Work out the finished part from the listing and answer in its coordinate system (mm). A direction names the side the tool comes from. Round coordinates to 2 decimals unless told otherwise and drop trailing zeros. Order: outer loops, then holes, each group sorted by start corner. A loop starts at its lowest first (then second) coordinate and runs counter-clockwise, first axis right, second up. Notation, with made-up numbers: M 33.5,-10 L 82.5,-10 A25 ccw 82.5,17 Z; hole C 59,62.5 d10. An arc over 180 degrees is marked long. Return JSON: item names as keys, results as strings.
from build123d import *

# Parameters (mm, degrees)
SALIENTE_EXTRUIR1_DEPTH = 1.8
CROQUIS2_W              = 7.6
CROQUIS2_H              = 25
SALIENTE_EXTRUIR2_DEPTH = 0.9
SALIENTE_EXTRUIR3_DEPTH = 3
CORTAR_EXTRUIR1_DEPTH   = 2.05
SALIENTE_EXTRUIR4_DEPTH = 20
REDONDEO1_R             = 2


with BuildPart() as part:
    # Croquis1 → Saliente-Extruir1 (new body)
    with BuildSketch(Plane.XY):
        Polygon((0, 0), (25, 0), (0, -25), align=None)
    extrude(amount=SALIENTE_EXTRUIR1_DEPTH)

    # Croquis2 → Saliente-Extruir2 (add)
    with BuildSketch(Plane.ZY):
        with Locations((-2, -12.5)):
            Rectangle(CROQUIS2_W, CROQUIS2_H)
    extrude(amount=SALIENTE_EXTRUIR2_DEPTH)

    # Croquis3 → Saliente-Extruir3 (add)
    with BuildSketch(Plane(origin=(0, 0, -5.8), x_dir=(-1, 0, 0), z_dir=(0, 0, -1))):
        Polygon((0, 0), (-25, 0), (0, -25), align=None)
    extrude(amount=-SALIENTE_EXTRUIR3_DEPTH)

    # Croquis4 → Cortar-Extruir1 (cut)
    with BuildSketch(Plane.XY.offset(-2.8)):
        Polygon((18.8816387, -4.704147737), (4.704147737, -18.8816387), (0.426151711, -14.603642674), (14.603642674, -0.426151711), align=None)
    extrude(amount=-CORTAR_EXTRUIR1_DEPTH, mode=Mode.SUBTRACT)

    # Croquis5 → Saliente-Extruir4 (add)
    with BuildSketch(Plane.ZY.offset(0.9)):
        Polygon((1.8, 0), (7.8, 0), (9.921320344, -2.121320344), (9.072792206, -2.969848481), (7.302943725, -1.2), (1.8, -1.2), align=None)
    extrude(amount=-SALIENTE_EXTRUIR4_DEPTH)

    # Redondeo1
    redondeo1_edges = [part.edges().sort_by_distance(p)[0] for p in [
        (9.1, 0, 7.8),
        (9.1, -1.2, 7.302943725),
    ]]
    fillet(redondeo1_edges, radius=REDONDEO1_R)


solid = part.part
Item 1: Which of the six approach directions +Z, -Z, +X, -X, +Y, -Y give full straight-line access (tool end or side, diameter ignored) to faces 1 (the flat face through (8.96, -2.386, 8.489)), 2 (the flat face through (0, -12, -1)), 3 (the flat face through (13, -12, -4)), 4 (the flat face through (7.42, -7.61, -3.81))?
Output:
{"face 1": "+X, -X, -Y", "face 2": "+X, +Y, -Y", "face 3": "+Z, -Z, +X, -Y", "face 4": "none"}
Item 2: Find section C-C (y = -21). Determine the outline of the cut face in (x, z).
Output:
{"outline": "M -0.9,-5.8 L 4,-5.8 L 4,-2.8 L 0,-2.8 L 0,0 L 4,0 L 4,1.8 L -0.9,1.8 Z"}
Item 3: Find section D-D (x = 22.75). Determine the outline of the cut face in (y, z), plus the area to 3 significant figures.
Output:
{"outline": "M -2.25,-5.8 L 0,-5.8 L 0,-2.8 L -2.25,-2.8 Z; M -2.25,0 L 0,0 L 0,1.8 L -2.25,1.8 Z", "area": "10.8 mm^2"}
Item 4: Find section A-A (x = 20). Determine the outline of the cut face in (y, z), plus the area to 3 significant figures.
Output:
{"outline": "M -5,-5.8 L 0,-5.8 L 0,-2.8 L -5,-2.8 Z; M -5,0 L 0,0 L 0,1.8 L -5,1.8 Z", "area": "24.0 mm^2"}
Item 5: The mould has two halves that part along Y. Classify faces 5 (the flat face through (19.1, -1, 6)), 6 (the flat face through (11.892, -11.694, -3.811)), 7 (the cylindrical face through (9.24, -0.15, 7.73)): pulls with the +Y half, pulls with the -Y half, needs draft (parallel to the pull), parting line crosses it, or undercut.
Output:
{"face 5": "needs draft", "face 6": "undercut", "face 7": "pulls with the +Y half"}
Item 6: Find section B-B (z = -4.5). Determine the outline of the cut face in (x, y).
Output:
{"outline": "M -0.9,-25 L 0,-25 L 25,0 L -0.9,0 Z; hole M 0.43,-14.6 L 4.7,-18.88 L 18.88,-4.7 L 14.6,-0.43 Z"}
Item 7: Each of these flat-tipped pins is pushed along its axis until it touches: pin 1 (5 mm diameter, centred on x = 4, y = -13, fed in from +Z); pin 2 (1.5 mm diameter, centred on x = 5, z = -3.5, fed in from -Y); pin 3 (12.5 mm diameter, centred on x = 18.5, y = -11, fed in from -Z); pin 4 (2.5 mm diameter, centred on x = 8, z = 4, fed in from -Y). Where does it stop, or does it pass through?
Output:
{"pin 1": "stops at z = 1.8", "pin 2": "stops at y = -20.75", "pin 3": "stops at z = -5.8", "pin 4": "stops at y = -1.2"}
Item 8: Consider line 1 along Z through (x, y) = (1.75, -17.75); line 2 along Z through (x, y) = (9.25, -12); line 3 along Z through (x, y) = (4.5, -2.75). Determine where each line is inside the solid, lowest interval first. Write a range as [from, to].
Output:
{"line 1": "z = [-5.8, -2.8], [0, 1.8]", "line 2": "z = [-5.8, -4.85], [0, 1.8]", "line 3": "z = [-5.8, -2.8], [0, 1.8], [8.85, 9.29]"}
